```python
from build123d import *

# Parameters (mm, degrees)
SKETCH1_W           = 6.8
SKETCH1_H           = 6.8
SKETCH1_R           = 1.75
BOSS_EXTRUDE1_DEPTH = 50
CUT_EXTRUDE1_DEPTH  = 8
SKETCH5_W           = 6.8
SKETCH5_H           = 6.8
BOSS_EXTRUDE2_DEPTH = 7
SKETCH3_W           = 6.8
SKETCH3_H           = 3.8
CUT_EXTRUDE2_DEPTH  = 15
SKETCH4_R           = 2.5
CUT_EXTRUDE3_DEPTH  = 20
FILLET3_RADIUS      = 3.4
FILLET3_LENGTH      = 3


with BuildPart() as part:
    # Sketch1 → Boss-Extrude1 (new body)
    with BuildSketch(Plane.XY):
        with Locations((-3.4, 3.4)):
            Rectangle(SKETCH1_W, SKETCH1_H)
        with Locations((-3.4, 3.4)):
            Circle(SKETCH1_R, mode=Mode.SUBTRACT)
    extrude(amount=BOSS_EXTRUDE1_DEPTH)

    # Sketch2 → Cut-Extrude1 (cut)
    with BuildSketch(Plane(origin=(0, 0, 0), x_dir=(-1, 0, 0), z_dir=(0, 0, -1))):
        Polygon((6.575426481, 3.4), (4.98771324, 6.15), (1.81228676, 6.15), (0.224573519, 3.4), (1.81228676, 0.65), (4.98771324, 0.65), align=None)
    extrude(amount=-CUT_EXTRUDE1_DEPTH, mode=Mode.SUBTRACT)

    # Sketch5 → Boss-Extrude2 (add)
    with BuildSketch(Plane.XY.offset(50)):
        with Locations((-3.4, 3.4)):
            Rectangle(SKETCH5_W, SKETCH5_H)
    extrude(amount=-BOSS_EXTRUDE2_DEPTH)

    # Sketch3 → Cut-Extrude2 (cut)
    with BuildSketch(Plane.XY.offset(50)):
        with Locations((-3.4, 1.9)):
            Rectangle(SKETCH3_W, SKETCH3_H)
    extrude(amount=-CUT_EXTRUDE2_DEPTH, mode=Mode.SUBTRACT)

    # Sketch4 → Cut-Extrude3 (cut)
    with BuildSketch(Plane.XZ.offset(-3.8)):
        with Locations((-3.4, 46.6)):
            Circle(SKETCH4_R)
    extrude(amount=-CUT_EXTRUDE3_DEPTH, mode=Mode.SUBTRACT)

    # Fillet3: full round fillet: the end face becomes a half cylinder, R = half its width
    fillet3_face = Plane((-3.4, 5.3, 50), x_dir=(0, -1, 0), z_dir=(0, 0, 1))  # on the end face: x along it, z out of the body
    fillet3_slab = fillet3_face.offset(-FILLET3_RADIUS / 2) * Box(FILLET3_LENGTH, 2 * FILLET3_RADIUS, FILLET3_RADIUS, mode=Mode.PRIVATE)  # the body's end, R deep
    fillet3_round = Plane((-3.4, 5.3, 46.6), x_dir=(0, 0, 1), z_dir=(0, -1, 0)) * Cylinder(FILLET3_RADIUS, FILLET3_LENGTH, mode=Mode.PRIVATE)  # its axis R under the face
    add(fillet3_slab - fillet3_round, mode=Mode.SUBTRACT)


solid = part.part
```
Can you work these out from the model? Positions are in its coordinate system, mm. A direction names the side the tool comes from. Coordinates: 2 decimals unless noted, no trailing zeros. Loops run counter-clockwise (first coordinate to the right, second up) from the corner with the lowest first, then second, coordinate; pieces in that order, holes last. Notation, with made-up numbers: (16.5, -36.5) - (69.5, -36.5) arc R13 cw to (69.5, -16.5) - close; hole circle Ø8 at (34.5, 34.5). An arc over 180 degrees is marked (long way). Use a Markdown table: item, result.
Item 1: I want a section at C-C on y = 2.75. Please give me the cut outline in (x, z).
Numbers:
| item | result |
|---|---|
| outline | (-6.8, 0) - (-6.2, 0) - (-6.2, 8) - (-5.02, 8) - (-5.02, 35) - (-6.8, 35) - close; (-1.78, 8) - (-0.6, 8) - (-0.6, 0) - (0, 0) - (0, 35) - (-1.78, 35) - close |
Item 2: I want a section at B-B on z = 7. Please give me the cut outline in (x, y), and give its area (3 significant figures).
Numbers:
| item | result |
|---|---|
| outline | (-6.8, 0) - (0, 0) - (0, 6.8) - (-6.8, 6.8) - close; hole (-6.58, 3.4) - (-4.99, 0.65) - (-1.81, 0.65) - (-0.22, 3.4) - (-1.81, 6.15) - (-4.99, 6.15) - close |
| area | 20.0 mm2 |
Item 3: We'd pull the mould along X, two halves only. Please class faces 5 (the face through (-3.45, 1.5, 35)), 6 (the face through (-1.03, 4.794, 3.944)), 7 (the face through (-3.3, 5.3, 50)): released by +X, released by -X, zero draft, split by the parting line, or undercut.
Numbers:
| item | result |
|---|---|
| face 5 | zero draft |
| face 6 | undercut |
| face 7 | split by the parting line |
Item 4: I want a section at A-A on x = -3.4. Please give me the cut outline in (y, z).
Numbers:
| item | result |
|---|---|
| outline | (0, 0) - (0.65, 0) - (0.65, 8) - (1.65, 8) - (1.65, 35) - (0, 35) - close; (3.8, 43) - (5.15, 43) - (5.15, 8) - (6.15, 8) - (6.15, 0) - (6.8, 0) - (6.8, 44.1) - (3.8, 44.1) - close; (3.8, 49.1) - (6.8, 49.1) - (6.8, 50) - (3.8, 50) - close |
Item 5: If I drill on probe 1 along Y at (x, z) = (-3.4, 18); probe 2 along X at (y, z) = (3.4, 22.5); probe 3 along Z at (x, y) = (-3.4, 4.9), over which ranges is the centre line in solid material (lowest first)? Write a range as from..to.
Numbers:
| item | result |
|---|---|
| probe 1 | y = 0..1.65, 5.15..6.8 |
| probe 2 | x = -6.8..-5.15, -1.65..0 |
| probe 3 | z = 43..44.1, 49.1..50 |
Item 6: For faces 1 (the face through (-3, 4, 43)), 2 (the face through (-5, 5, 8)), 3 (the face through (-6, 3.8, 43)), 4 (the face through (-6.8, 3, 23)), which set-ups out of +Z, -Z, +X, -X, +Y, -Y let a thin tool reach every point of the face, with its end or its side?
Numbers:
| item | result |
|---|---|
| face 1 | -Z, -Y |
| face 2 | -Z |
| face 3 | +Z, +X, -X, -Y |
| face 4 | +Z, -Z, -X, +Y, -Y |
Item 7: I want a section at D-D on z = 42. Please give me the cut outline in (x, y), and give its area (3 significant figures).
Numbers:
| item | result |
|---|---|
| outline | (-6.8, 3.8) - (-5.1, 3.8) arc R1.75 cw to (-1.7, 3.8) - (0, 3.8) - (0, 6.8) - (-6.8, 6.8) - close |
| area | 17.0 mm2 |
Item 8: Will these pins go through, and if not, where does the flat tip stop? pin 1 (4 mm diameter, centred on x = -5, y = 4.5, fed in from -Z); pin 2 (1.1 mm diameter, centred on x = -3, y = 2, fed in from +Z); pin 3 (4 mm diameter, centred on x = -3.4, z = 46.6, fed in from +Y); pin 4 (3 mm diameter, centred on x = -6, y = 4.5, fed in from +Z).
Numbers:
| item | result |
|---|---|
| pin 1 | stops at z = 0 |
| pin 2 | stops at z = 35 |
| pin 3 | passes through |
| pin 4 | stops at z = 49.82 |
